Work out the finished part from the listing and answer in its coordinate system (mm). A direction names the side the tool comes from. Round coordinates to 2 decimals unless told otherwise and drop trailing zeros. Loops run counter-clockwise (first coordinate to the right, second up) from the corner with the lowest first, then second, coordinate; pieces in that order, holes last.
```python
from build123d import *

# Parameters (mm, degrees)
F3_DEPTH = 1


with BuildPart() as f1:
    # F0 (on Right) → F1 (revolve)
    with BuildSketch(Plane.YZ):
        with BuildLine():
            Line((-61.0699225962, 0), (-22.4797911942, 0))
            Line((-22.4797911942, 0), (-11.0699225962, 38))
            ThreePointArc((-11.0699225962, 38), (-7.5699225962, 41.5), (-11.0699225962, 45))
            Line((-11.0699225962, 45), (-8.0699225962, 45))
            Line((-8.0699225962, 45), (-8.0699225962, 49))
            Line((-8.0699225962, 49), (-7.5699225962, 49))
            Line((-7.5699225962, 49), (-7.5699225962, 50))
            Line((-7.5699225962, 50), (-13.0699225962, 50))
            Line((-13.0699225962, 50), (-13.0699225962, 45))
            Line((-13.0699225962, 45), (-16.0699225962, 45))
            Line((-16.0699225962, 45), (-36.0699225962, 37.823528317))
            Line((-36.0699225962, 37.823528317), (-36.0699225962, 33.2837096231))
            Line((-36.0699225962, 33.2837096231), (-41.0699225962, 31.4013561058))
            Line((-41.0699225962, 31.4013561058), (-41.0699225962, 36))
            Line((-41.0699225962, 36), (-61.0699225962, 36))
            Line((-61.0699225962, 36), (-61.0699225962, 0))
        make_face()
    revolve(axis=Axis((0, -30.5349612981, 0), (0, -1, 0)))

    # F2 (on face) → F3 (join)
    with BuildSketch(Plane.XZ.offset(13.0699225962)):
        with BuildLine():
            Line((12.8560631669, 48.3189573547), (4.4851679108, 62.2098119404))
            Line((4.4851679108, 62.2098119404), (4.04924654, 62.9331898094))
            ThreePointArc((4.04924654, 62.9331898094), (0, 65), (-4.04924654, 62.9331898094))
            Line((-4.04924654, 62.9331898094), (-4.4851679108, 62.2098119404))
            Line((-4.4851679108, 62.2098119404), (-12.8560631669, 48.3189573547))
            ThreePointArc((-12.8560631669, 48.3189573547), (0, 50), (12.8560631669, 48.3189573547))
        make_face()
        with BuildLine():
            ThreePointArc((2.4997371633, 59.536250715), (2.5, 59.5), (2.4997371633, 59.463749285))
            Line((2.4997371633, 59.463749285), (2.4997371633, 57.536250715))
            ThreePointArc((2.4997371633, 57.536250715), (2.5, 57.5), (2.4997371633, 57.463749285))
            ThreePointArc((2.4997371633, 57.463749285), (0.0126154042, 55.0000318299), (-2.4992440087, 57.4385232966))
            ThreePointArc((-2.4992440087, 57.4385232966), (-2.5, 57.5), (-2.4992440087, 57.5614767034))
            Line((-2.4992440087, 57.5614767034), (-2.4992440087, 59.4385232966))
            ThreePointArc((-2.4992440087, 59.4385232966), (-2.5, 59.5), (-2.4992440087, 59.5614767034))
            ThreePointArc((-2.4992440087, 59.5614767034), (0.0126154042, 61.9999681701), (2.4997371633, 59.536250715))
        make_face(mode=Mode.SUBTRACT)
        with BuildLine():
            Line((62.2098119404, 4.4851679108), (48.3189573547, 12.8560631669))
            ThreePointArc((48.3189573547, 12.8560631669), (49.5779581454, 6.4827514322), (50, 0))
            ThreePointArc((50, 0), (49.5779581454, -6.4827514322), (48.3189573547, -12.8560631669))
            Line((48.3189573547, -12.8560631669), (62.2098119404, -4.4851679108))
            Line((62.2098119404, -4.4851679108), (62.9331898094, -4.04924654))
            ThreePointArc((62.9331898094, -4.04924654), (65, 0), (62.9331898094, 4.04924654))
            Line((62.9331898094, 4.04924654), (62.2098119404, 4.4851679108))
        make_face()
        with BuildLine():
            ThreePointArc((57.4385232966, 2.4992440087), (57.5, 2.5), (57.5614767034, 2.4992440087))
            Line((57.5614767034, 2.4992440087), (59.4385232966, 2.4992440087))
            ThreePointArc((59.4385232966, 2.4992440087), (59.5, 2.5), (59.5614767034, 2.4992440087))
            ThreePointArc((59.5614767034, 2.4992440087), (61.9999681701, -0.0126154042), (59.536250715, -2.4997371633))
            ThreePointArc((59.536250715, -2.4997371633), (59.5, -2.5), (59.463749285, -2.4997371633))
            Line((59.463749285, -2.4997371633), (57.536250715, -2.4997371633))
            ThreePointArc((57.536250715, -2.4997371633), (57.5, -2.5), (57.463749285, -2.4997371633))
            ThreePointArc((57.463749285, -2.4997371633), (55.0000318299, -0.0126154042), (57.4385232966, 2.4992440087))
        make_face(mode=Mode.SUBTRACT)
        with BuildLine():
            ThreePointArc((-48.3189573547, -12.8560631669), (-50, 0), (-48.3189573547, 12.8560631669))
            Line((-48.3189573547, 12.8560631669), (-62.2098119404, 4.4851679108))
            Line((-62.2098119404, 4.4851679108), (-62.9331898094, 4.04924654))
            ThreePointArc((-62.9331898094, 4.04924654), (-65, 0), (-62.9331898094, -4.04924654))
            Line((-62.9331898094, -4.04924654), (-62.2098119404, -4.4851679108))
            Line((-62.2098119404, -4.4851679108), (-48.3189573547, -12.8560631669))
        make_face()
        with BuildLine():
            ThreePointArc((-57.4385232966, -2.4992440087), (-57.5, -2.5), (-57.5614767034, -2.4992440087))
            Line((-57.5614767034, -2.4992440087), (-59.4385232966, -2.4992440087))
            ThreePointArc((-59.4385232966, -2.4992440087), (-59.5, -2.5), (-59.5614767034, -2.4992440087))
            ThreePointArc((-59.5614767034, -2.4992440087), (-61.9999681701, 0.0126154042), (-59.536250715, 2.4997371633))
            ThreePointArc((-59.536250715, 2.4997371633), (-59.5, 2.5), (-59.463749285, 2.4997371633))
            Line((-59.463749285, 2.4997371633), (-57.536250715, 2.4997371633))
            ThreePointArc((-57.536250715, 2.4997371633), (-57.5, 2.5), (-57.463749285, 2.4997371633))
            ThreePointArc((-57.463749285, 2.4997371633), (-55.0000318299, 0.0126154042), (-57.4385232966, -2.4992440087))
        make_face(mode=Mode.SUBTRACT)
        with BuildLine():
            Line((4.4851679108, -62.2098119404), (12.8560631669, -48.3189573547))
            ThreePointArc((12.8560631669, -48.3189573547), (0, -50), (-12.8560631669, -48.3189573547))
            Line((-12.8560631669, -48.3189573547), (-4.4851679108, -62.2098119404))
            Line((-4.4851679108, -62.2098119404), (-4.04924654, -62.9331898094))
            ThreePointArc((-4.04924654, -62.9331898094), (0, -65), (4.04924654, -62.9331898094))
            Line((4.04924654, -62.9331898094), (4.4851679108, -62.2098119404))
        make_face()
        with BuildLine():
            ThreePointArc((2.4992440087, -57.4385232966), (2.5, -57.5), (2.4992440087, -57.5614767034))
            Line((2.4992440087, -57.5614767034), (2.4992440087, -59.4385232966))
            ThreePointArc((2.4992440087, -59.4385232966), (2.5, -59.5), (2.4992440087, -59.5614767034))
            ThreePointArc((2.4992440087, -59.5614767034), (-0.0126154042, -61.9999681701), (-2.4997371633, -59.536250715))
            ThreePointArc((-2.4997371633, -59.536250715), (-2.5, -59.5), (-2.4997371633, -59.463749285))
            Line((-2.4997371633, -59.463749285), (-2.4997371633, -57.536250715))
            ThreePointArc((-2.4997371633, -57.536250715), (-2.5, -57.5), (-2.4997371633, -57.463749285))
            ThreePointArc((-2.4997371633, -57.463749285), (-0.0126154042, -55.0000318299), (2.4992440087, -57.4385232966))
        make_face(mode=Mode.SUBTRACT)
    extrude(amount=-F3_DEPTH)


solid = f1.part
```
1. Given pin 1 (8.5 mm diameter, centred on x = -57.5, z = 4.5, fed in from +Y); pin 2 (8 mm diameter, centred on y = -38, z = 25.5, fed in from -X); pin 3 (1.1 mm diameter, centred on x = -58.5, y = -12.5, fed in from +Z), each flat-ended and moving along its own axis, determine where each tip first touches the part or whether it passes through.
Answer key:
pin 1: stops at y = -12.07
pin 2: stops at x = -30.77
pin 3: stops at z = 7.05
2. Consider probe 1 along Z at (x, y) = (0, -7.9); probe 2 along Z at (x, y) = (0, -9.9); probe 3 along X at (y, z) = (-9.05, 0). Determine where each line is inside the solid, lowest interval first.
Answer key:
probe 1: z = -50 to -49, -42.98 to -40.02, 40.02 to 42.98, 49 to 50
probe 2: z = -50 to -45, -44.8 to -38.2, 38.2 to 44.8, 45 to 50
probe 3: x = -50 to -45, -44.36 to -38.64, 38.64 to 44.36, 45 to 50
3. Find section C-C (y = -34). Write down the section's boundary in (x, z).
Answer key:
outline: circle Ø77.13 at (0, 0)
4. Find section A-A (y = -54.5). Write down the section's boundary in (x, z).
Answer key:
outline: circle Ø72 at (0, 0)
5. Find section B-B (y = -18). Write down the section's boundary in (x, z), then the cut area to 3 significant figures.
Answer key:
outline: circle Ø88.61 at (0, 0); hole circle Ø29.84 at (0, 0)
area: 5,470 mm2
6. Determine the mould class of faces 1 (the face through (-41.32, -7.82, 26.34)), 2 (the face through (-9.46, -40.827, 30.038)), 3 (the face through (-11.5, -35.1, 36.4)), 4 (the face through (33.44, -36.07, -0.18)) for opening direction Y: +Y half, -Y half, draft (parallel to the pull), parting line (faces both ways), or undercut.
Answer key:
face 1: draft
face 2: undercut
face 3: -Y half
face 4: undercut
7. Which of the six approach directions +Z, -Z, +X, -X, +Y, -Y give full straight-line access (tool end or side, diameter ignored) to faces 5 (the face through (14, -13.07, -43)), 6 (the face through (40, -8.07, -22)), 7 (the face through (-30, -41.07, 11)), 8 (the face through (-1, -61.07, -1))?
Answer key:
face 5: -Y
face 6: +Y
face 7: none
face 8: +Z, -Z, +X, -X, -Y
